Here's how the part is built. I have some questions about the finished solid (model axes, mm). A direction names the side the tool comes from. Coordinates: 2 decimals unless noted, no trailing zeros. Order: outer loops, then holes, each group sorted by start corner. A loop starts at its lowest first (then second) coordinate and runs counter-clockwise, first axis right, second up. Notation, with made-up numbers: (53.25, -34.5) - (105.25, -34.5) arc R31 cw to (105.25, 4.5) - close; hole circle Ø6 at (77.25, -16.75). An arc over 180 degrees is marked (long way). Answer as CSV lines item,"result". Start each with the question number.
Item 1: Imagine slicing it at A-A on x = 8. List the corners of the cut face in (y, z) for me.
Item 2: Imagine slicing it at D-D on x = 89.5. List the corners of the cut face in (y, z) for me, and give its area (3 significant figures).
Item 3: I'm going to push flat-ended pins straight in: pin 1 (3.5 mm diameter, centred on x = 76, z = -57.5, fed in from -Y); pin 2 (2 mm diameter, centred on x = 9.5, z = -57, fed in from +Y); pin 3 (6 mm diameter, centred on x = 92, z = -8, fed in from -Y); pin 4 (2 mm diameter, centred on y = 2, z = -1, fed in from -X). Where does each tip first touch, or does it pass through?
Item 4: Imagine slicing it at B-B on z = -57.5. List the corners of the cut face in (x, y) for me, and give its area (3 significant figures).
Item 5: Imagine slicing it at C-C on z = -8. List the corners of the cut face in (x, y) for me.
Item 6: We'd pull the mould along X, two halves only. Please class faces 1 (the face through (100, 3, -33)), 2 (the face through (97, 2, -62)), 3 (the face through (18.601, 4.768, -55.592)), 4 (the face through (98, 2, -33)): pulls with the +X half, pulls with the -X half, needs draft (parallel to the pull), parting line crosses it, or undercut.
Item 7: On a 3-axis mill with a long thin cutter (end or side, diameter ignored), from which of +Z, -Z, +X, -X, +Y, -Y can I reach the whole of each face in a straight line? I mean faces 5 (the face through (89.7, 4.9, -60.9)), 6 (the face through (1, 2, -61)), 7 (the face through (4, 2, -3)), 8 (the face through (51, 2, -64)), 9 (the face through (51, 3, -66)). Say none if no direction works.
Item 8: I need wall thicknesses on line 1 (X direction, y = 4.2, z = -8.5); line 2 (X direction, y = 4.9, z = -58); line 3 (Z direction, x = 95, y = 2.9). Which ranges of each line are inside material? Lowest first, please.
from build123d import *

# Parameters (mm, degrees)
BOSS_EXTRUDE2_DEPTH = 6
CUT_EXTRUDE1_DEPTH  = 3.5
SKETCH5_R           = 3.7
CUT_EXTRUDE2_DEPTH  = 2.2
SKETCH6_R           = 2
CUT_EXTRUDE3_DEPTH  = 120.966662036
SKETCH11_W          = 2.417424305
SKETCH11_H          = 56
SKETCH11_W_2        = 86.709228263
SKETCH11_H_2        = 2
CUT_EXTRUDE7_DEPTH  = 3.5


with BuildPart() as part:
    # Sketch1 → Boss-Extrude2 (new body)
    with BuildSketch(Plane(origin=(0, 0, 0), x_dir=(1, 0, 0), z_dir=(0, 1, 0))):
        with BuildLine():
            Line((5, 0), (95, 0))
            ThreePointArc((95, 0), (98.535533906, 1.464466094), (100, 5))
            Line((100, 5), (100, 61))
            ThreePointArc((100, 61), (98.535533906, 64.535533906), (95, 66))
            Line((95, 66), (5, 66))
            ThreePointArc((5, 66), (1.464466094, 64.535533906), (0, 61))
            Line((0, 61), (0, 5))
            ThreePointArc((0, 5), (1.464466094, 1.464466094), (5, 0))
        make_face()
    extrude(amount=BOSS_EXTRUDE2_DEPTH)

    # Sketch2 → Cut-Extrude1 (cut)
    with BuildSketch(Plane.XZ):
        with BuildLine():
            Line((7, -2), (93, -2))
            ThreePointArc((93, -2), (96.535533906, -3.464466094), (98, -7))
            Line((98, -7), (98, -59))
            ThreePointArc((98, -59), (96.535533906, -62.535533906), (93, -64))
            Line((93, -64), (7, -64))
            ThreePointArc((7, -64), (3.464466094, -62.535533906), (2, -59))
            Line((2, -59), (2, -7))
            ThreePointArc((2, -7), (3.464466094, -3.464466094), (7, -2))
        make_face()
    extrude(amount=-CUT_EXTRUDE1_DEPTH, mode=Mode.SUBTRACT)

    # Sketch5 → Cut-Extrude2 (cut)
    with BuildSketch(Plane(origin=(0, 6, 0), x_dir=(1, 0, 0), z_dir=(0, 1, 0))):
        with Locations(Location((8, 58, 0), (0, 0, 270))):
            Circle(SKETCH5_R)
        with Locations(Location((8, 8, 0), (0, 0, 270))):
            Circle(SKETCH5_R)
        with Locations(Location((92, 58, 0), (0, 0, 270))):
            Circle(SKETCH5_R)
        with Locations(Location((92, 8, 0), (0, 0, 270))):
            Circle(SKETCH5_R)
    extrude(amount=-CUT_EXTRUDE2_DEPTH, mode=Mode.SUBTRACT)

    # Sketch6 → Cut-Extrude3 (cut, through all)
    with BuildSketch(Plane(origin=(0, 6, 0), x_dir=(1, 0, 0), z_dir=(0, 1, 0))):
        with Locations(Location((18, 57.5, 0), (0, 0, 270))):
            Circle(SKETCH6_R)
        with Locations(Location((18, 8.5, 0), (0, 0, 270))):
            Circle(SKETCH6_R)
        with Locations(Location((76, 57.5, 0), (0, 0, 270))):
            Circle(SKETCH6_R)
        with Locations(Location((76, 8.5, 0), (0, 0, 270))):
            Circle(SKETCH6_R)
    extrude(amount=-CUT_EXTRUDE3_DEPTH, mode=Mode.SUBTRACT)

    # Sketch11 → Cut-Extrude7 (cut)
    with BuildSketch(Plane(origin=(0, 0, 0), x_dir=(-1, 0, 0), z_dir=(0, -1, 0))):
        with Locations((-1.208712152, 33)):
            Rectangle(SKETCH11_W, SKETCH11_H)
        with Locations((-49.645385869, 1)):
            Rectangle(SKETCH11_W_2, SKETCH11_H_2)
    extrude(amount=-CUT_EXTRUDE7_DEPTH, mode=Mode.SUBTRACT)


solid = part.part
Responses:
1,outline,"(0, -66) - (6, -66) - (6, -61.7) - (3.8, -61.7) - (3.8, -54.3) - (6, -54.3) - (6, -11.7) - (3.8, -11.7) - (3.8, -4.3) - (6, -4.3) - (6, 0) - (3.5, 0) - (3.5, -64) - (0, -64) - close"
2,outline,"(0, -66) - (6, -66) - (6, -60.73) - (3.8, -60.73) - (3.8, -55.27) - (6, -55.27) - (6, -10.73) - (3.8, -10.73) - (3.8, -5.27) - (6, -5.27) - (6, 0) - (3.5, 0) - (3.5, -64) - (0, -64) - close"
2,area,"148 mm^2"
3,pin 1,"passes through"
3,pin 2,"stops at y = 3.8"
3,pin 3,"stops at y = 3.5"
3,pin 4,"stops at x = 1"
4,outline,"(0, 3.5) - (16, 3.5) - (16, 6) - (11.67, 6) - (11.67, 3.8) - (4.33, 3.8) - (4.33, 6) - (0, 6) - close; (20, 3.5) - (74, 3.5) - (74, 6) - (20, 6) - close; (78, 3.5) - (98, 3.5) - (98, 0) - (100, 0) - (100, 6) - (95.67, 6) - (95.67, 3.8) - (88.33, 3.8) - (88.33, 6) - (78, 6) - close"
4,area,"205 mm^2"
5,outline,"(0, 3.5) - (16.06, 3.5) - (16.06, 6) - (11.7, 6) - (11.7, 3.8) - (4.3, 3.8) - (4.3, 6) - (0, 6) - close; (19.94, 3.5) - (74.06, 3.5) - (74.06, 6) - (19.94, 6) - close; (77.94, 3.5) - (98, 3.5) - (98, 0) - (100, 0) - (100, 6) - (95.7, 6) - (95.7, 3.8) - (88.3, 3.8) - (88.3, 6) - (77.94, 6) - close"
6,face 1,"pulls with the +X half"
6,face 2,"undercut"
6,face 3,"undercut"
6,face 4,"pulls with the -X half"
7,face 5,"+Y"
7,face 6,"-X, -Y"
7,face 7,"-Y"
7,face 8,"+Z, -Y"
7,face 9,"-Z, +X, -X, +Y, -Y"
8,line 1,"x = 0 to 4.33, 11.67 to 16, 20 to 74, 78 to 88.33, 95.67 to 100"
8,line 2,"x = 0 to 4.3, 11.7 to 16.06, 19.94 to 74.06, 77.94 to 88.3, 95.7 to 100"
8,line 3,"z = -66 to -63.58, -2.42 to 0"
